Can you work these out from the model? Positions are in its coordinate system, mm. Coordinates: 2 decimals unless noted, no trailing zeros. Order: outer loops, then holes, each group sorted by start corner. A loop starts at its lowest first (then second) coordinate and runs counter-clockwise, first axis right, second up. Notation, with made-up numbers: (66.25, -14.5) -> (108.25, -14.5) arc R19 cw to (108.25, -5.5) -> close; hole circle Ø5 at (84.5, 22). An arc over 180 degrees is marked (long way). Return JSON: item names as keys, results as strings. Group by question number.
1) If I drill on probe 1 along X at (y, z) = (-6, 0); probe 2 along Z at (x, y) = (-135, -5); probe 3 along X at (y, z) = (-0.75, -13.5), over which ranges is the centre line in solid material (lowest first)? Write a range as from..to.
2) Thinking about a two-plate mould opening in X: for faces 1 (the cylindrical face through (-149.985, -4.93, 0.66)), 2 (the cylindrical face through (-164.297, -5.07, 31.486)), 3 (the flat face through (-2, -10, 1)), which applies, +X half, -X half, draft (parallel to the pull), parting line (faces both ways), or undercut?
3) If we section it at A-A, the plane z = -12: Please give me the cut outline in (x, y).
4) If we section it at D-D, the plane x = -143.5: Please give me the cut outline in (y, z).
5) If we section it at C-C, the plane y = -2.25: Please give me the cut outline in (x, z), then the cut area to 3 significant figures.
6) If we section it at B-B, the plane x = -25: Please give me the cut outline in (y, z).
from build123d import *

# Parameters (mm, degrees)
F0_W          = 340
F0_H          = 75
F1_DEPTH      = 10
F2_R          = 20
F3_R          = 15
F4_DEPTH      = 354
F4_DEPTH_BACK = 25


# Not quite as in the source:
# - an extrude ends at something that could not be found from the text; its depth is read off the source's solid


with BuildPart() as f1:
    # F0 (on Front) → F1 (new body)
    with BuildSketch(Plane.XZ):
        Rectangle(F0_W, F0_H)
    extrude(amount=F1_DEPTH)

    # F2
    f2_edges = [f1.edges().sort_by_distance(p)[0] for p in [
        (-170, -5, 37.5),
        (-170, -5, -37.5),
    ]]
    fillet(f2_edges, radius=F2_R)

    # F3 (on Front) → F4 (cut, two sides)
    with BuildSketch(Plane.XZ) as f4_sk:
        with Locations((-135, 0)):
            Circle(F3_R)
        with Locations((-25, 0)):
            Circle(F3_R)
    extrude(amount=-F4_DEPTH, mode=Mode.SUBTRACT)
    extrude(f4_sk.sketch, amount=F4_DEPTH_BACK, mode=Mode.SUBTRACT)


solid = f1.part
Result sheet:
{
 "1": {"probe 1": "x = -170..-150, -120..-40, -10..170", "probe 2": "z = -37.5..-15, 15..37.5", "probe 3": "x = -170..-141.54, -128.46..-31.54, -18.46..170"},
 "2": {"face 1": "undercut", "face 2": "-X half", "face 3": "draft"},
 "3": {"outline": "(-170, -10) -> (-144, -10) -> (-144, 0) -> (-170, 0) -> close; (-126, -10) -> (-34, -10) -> (-34, 0) -> (-126, 0) -> close; (-16, -10) -> (170, -10) -> (170, 0) -> (-16, 0) -> close"},
 "4": {"outline": "(-10, -37.5) -> (0, -37.5) -> (0, -12.36) -> (-10, -12.36) -> close; (-10, 12.36) -> (0, 12.36) -> (0, 37.5) -> (-10, 37.5) -> close"},
 "5": {"outline": "(-170, -17.5) arc R20 ccw to (-150, -37.5) -> (170, -37.5) -> (170, 37.5) -> (-150, 37.5) arc R20 ccw to (-170, 17.5) -> close; hole circle Ø30 at (-135, 0); hole circle Ø30 at (-25, 0)", "area": "23,900 mm2"},
 "6": {"outline": "(-10, -37.5) -> (0, -37.5) -> (0, -15) -> (-10, -15) -> close; (-10, 15) -> (0, 15) -> (0, 37.5) -> (-10, 37.5) -> close"}
}
